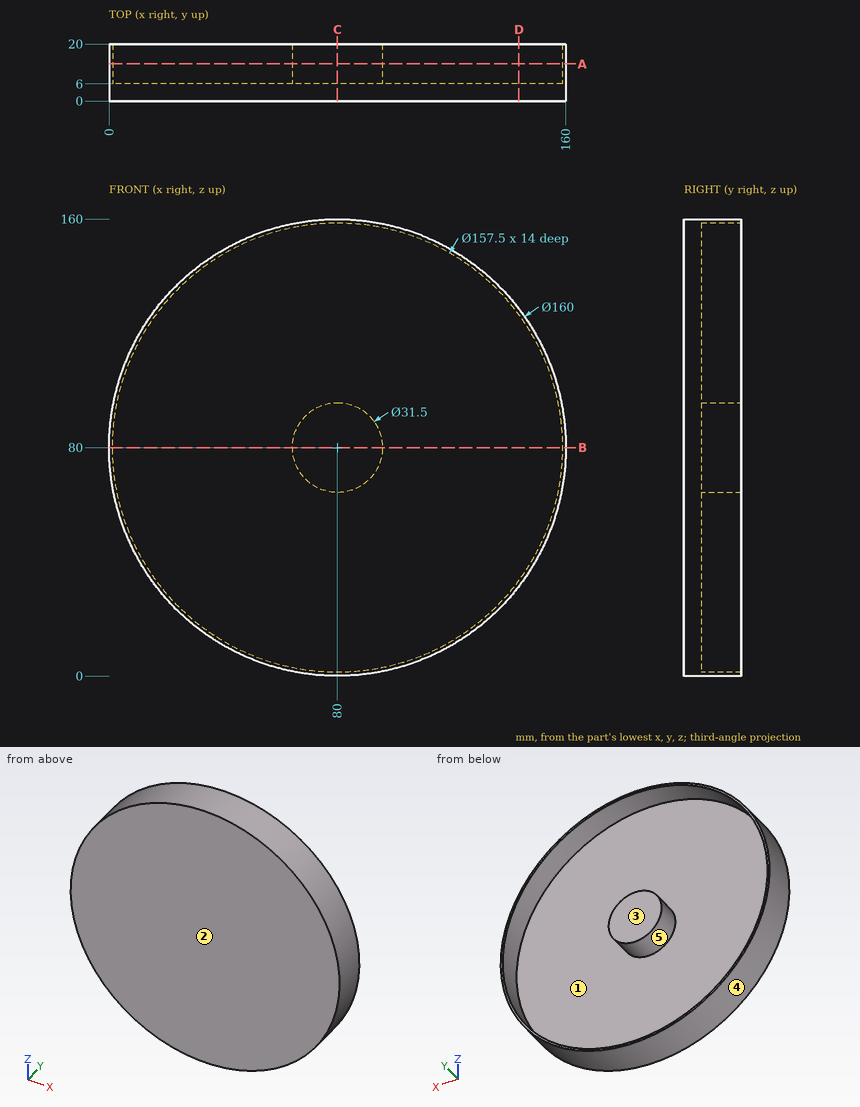
Source: three-view drawing plus pictorial views. Frame: mm from the lowest corner of the part. A direction names the side the tool comes from. Give positions to 0.01 mm unless a question says otherwise; leave off trailing zeros. Order: outer loops, then holes, each group sorted by start corner. A loop starts at its lowest first (then second) coordinate and runs counter-clockwise, first axis right, second up. Notation, with made-up numbers: (-28, 66) -> (31, 66) arc R24 ccw to (31, 89) -> close; hole circle Ø5 at (20, -28). An arc over 180 degrees is marked (long way). Write each question's results on one line, items separated by ' | '. Start each with the question number.
Item 1: Cut plane C-C on x = 80. Return the cut outline in (y, z).
Item 2: Mould query, pull axis Z, two halves, no side actions, for the marked faces 3, 4 and 5. Classes: pulls with the +Z half, pulls with the -Z half, needs draft (parallel to the pull), parting line crosses it, or undercut.
Item 3: Line query: line 1 (X direction, y = 12.5, z = 80); line 2 (Y direction, x = 30.5, z = 134); line 3 (X direction, y = 9, z = 117). Output: solid intervals per line, ascending.
Item 4: Cut plane A-A on y = 13. Return the cut outline in (x, z).
Item 5: Cut plane B-B on z = 80. Return the cut outline in (x, y), then the cut area to 3 significant figures.
Item 6: Set-up query: the marked faces 1 and 2. Return all of +Z, -Z, +X, -X, +Y, -Y with unobstructed straight access to the full face (end or side cutting, diameter ignored); none if empty.
Item 7: Contact query for flat-ended pins moving along their axis: P1, Ø5, axis at x = 58, y = 6.5, coming from the +Z side; P2, Ø2, axis at x = 141.5, y = 5.5, coming from the +Z side; P3, Ø4, axis at x = 134.5, z = 112.5, coming from the +Y side. Output: stop coordinate, or through.
Item 8: Cut plane D-D on x = 143.5. Return the cut outline in (y, z).
Established:
1) outline: (0, 0) -> (20, 0) -> (20, 1.25) -> (6, 1.25) -> (6, 64.25) -> (20, 64.25) -> (20, 95.75) -> (6, 95.75) -> (6, 158.75) -> (20, 158.75) -> (20, 160) -> (0, 160) -> close
2) face 3: needs draft | face 4: parting line crosses it | face 5: undercut
3) line 1: 0 to 1.25, 64.25 to 95.75, 158.75 to 160 | line 2: 0 to 6 | line 3: 9.07 to 10.48, 149.52 to 150.93
4) outline: circle Ø160 at (80, 80); circle Ø31.5 at (80, 80); hole circle Ø157.5 at (80, 80)
5) outline: (0, 0) -> (160, 0) -> (160, 20) -> (158.75, 20) -> (158.75, 6) -> (95.75, 6) -> (95.75, 20) -> (64.25, 20) -> (64.25, 6) -> (1.25, 6) -> (1.25, 20) -> (0, 20) -> close | area: 1,440 mm^2
6) face 1: +Y | face 2: +Z, -Z, +X, -X, -Y
7) P1: z = 157.59 | P2: z = 132.34 | P3: y = 6
8) outline: (0, 31.34) -> (20, 31.34) -> (20, 33.42) -> (6, 33.42) -> (6, 126.58) -> (20, 126.58) -> (20, 128.66) -> (0, 128.66) -> close
